Autodesk Inventor part; units mm, degrees
ref_plane "YZ Plane" through (0, 0, 0) normal (1, 0, 0) x (0, 1, 0)
ref_plane "XZ Plane" through (0, 0, 0) normal (0, 1, 0) x (-1, 0, 0)
ref_plane "XY Plane" through (0, 0, 0) normal (0, 0, 1) x (1, 0, 0)
sketch "Skizze1" plane through (0, 0, 0) normal (0, 1, 0) x (-1, 0, 0)
  line L0 (50.25, 43.85) -> (-50.25, 43.85)
  line L1 (-58.25, 35.85) -> (-58.25, -35.85)
  line L2 (-50.25, -43.85) -> (50.25, -43.85)
  line L3 (58.25, -35.85) -> (58.25, 35.85)
  line L4 (58.25, 43.85) -> (-58.25, -43.85) construction
  line L5 (-58.25, 43.85) -> (58.25, -43.85) construction
  arc A0 (58.25, 35.85) -> (50.25, 43.85) centre (50.25, 35.85) ccw
  arc A1 (50.25, -43.85) -> (58.25, -35.85) centre (50.25, -35.85) ccw
  arc A2 (-58.25, -35.85) -> (-50.25, -43.85) centre (-50.25, -35.85) ccw
  arc A3 (-50.25, 43.85) -> (-58.25, 35.85) centre (-50.25, 35.85) ccw
  point P0 (0, 0)
  dimension "d0" = 116.5
  dimension "d1" = 87.7
  dimension "d2" = 8
extrude "Extrusion1" add sketch "Skizze1" along normal blind 21
sketch "Skizze2" plane through (0, 0, 0) normal (0, -1, 0) x (1, 0, 0)
  arc A0 (58.25, 35.85) -> (50.25, 43.85) centre (50.25, 35.85) ccw
  line L0 (-50.25, 43.85) -> (50.25, 43.85)
  arc A1 (-50.25, 43.85) -> (-58.25, 35.85) centre (-50.25, 35.85) ccw
  line L1 (-58.25, -35.85) -> (-58.25, 35.85)
  arc A2 (-58.25, -35.85) -> (-50.25, -43.85) centre (-50.25, -35.85) ccw
  line L2 (50.25, -43.85) -> (-50.25, -43.85)
  arc A3 (50.25, -43.85) -> (58.25, -35.85) centre (50.25, -35.85) ccw
  line L3 (58.25, 35.85) -> (58.25, -35.85)
  line L4 (50.25, -43.85) -> (-50.25, -43.85)
  line L5 (-5.75, -43.85) -> (-5.75, 43.85)
  point P0 (0, 0)
  dimension "d5" = 64
extrude "Extrusion2" add sketch "Skizze2" along normal blind 0.1 contours L3 A3 L2 L5 L0 A0
sketch "Skizze3" plane through (0, 21, 0) normal (0, 1, 0) x (1, 0, 0)
  line L0 (-40.25, -30.75) -> (-2.65, -30.75)
  line L1 (-2.65, -30.75) -> (-2.65, 33.55)
  line L2 (-2.65, 33.55) -> (-40.25, 33.55)
  line L3 (-40.25, 33.55) -> (-40.25, -30.75)
  line L4 (-40.25, -30.75) -> (-2.65, 33.55) construction
  line L5 (-2.65, -30.75) -> (-40.25, 33.55) construction
  line L6 (-50.25, -43.85) -> (50.25, -43.85)
  line L7 (50.25, 43.85) -> (-50.25, 43.85)
  line L8 (-58.25, 35.85) -> (-58.25, -35.85)
  point P0 (0, 0)
  point P1 (-21.45, 1.4)
  dimension "d8" = 37.6
  dimension "d9" = 64.3
  dimension "d10" = 13.1
  dimension "d11" = 10.3
  dimension "d12" = 18
extrude "Extrusion3" add sketch "Skizze3" along normal blind 9
sketch "Skizze4" plane through (0, -0.1, 0) normal (0, -1, 0) x (1, 0, 0)
  line L0 (50.25, 43.85) -> (-5.75, 43.85)
  line L1 (-5.75, 43.85) -> (-5.75, -43.85)
  line L2 (-5.75, -43.85) -> (50.25, -43.85)
  arc A0 (50.25, -43.85) -> (58.25, -35.85) centre (50.25, -35.85) ccw
  line L3 (58.25, -35.85) -> (58.25, 35.85)
  arc A1 (58.25, 35.85) -> (50.25, 43.85) centre (50.25, 35.85) ccw
  line L4 (-5.75, -43.85) -> (-5.75, 43.85)
  line L5 (-50.25, 43.85) -> (-5.75, 43.85)
  arc A2 (-50.25, 43.85) -> (-58.25, 35.85) centre (-50.25, 35.85) ccw
  line L6 (-58.25, -35.85) -> (-58.25, 35.85)
  arc A3 (-58.25, -35.85) -> (-50.25, -43.85) centre (-50.25, -35.85) ccw
  line L7 (-5.75, -43.85) -> (-50.25, -43.85)
  circle A4 centre (43.75, -36.9) radius 1.1
  circle A5 centre (43.75, 29.95) radius 1.1
  circle A6 centre (-11.95, -35.9681) radius 1.1
  circle A7 centre (-8.45, 34.0319) radius 1.1
  circle A8 centre (-47.95, -34.8429) radius 1.1
  circle A9 centre (-53.15, 31.6571) radius 1.1
  point P0 (0, 0)
  dimension "d15" = 2.2
  dimension "d16" = 2.2
  dimension "d17" = 2.2
  dimension "d18" = 2.2
  dimension "d19" = 2.2
  dimension "d20" = 2.2
  dimension "d21" = 0
  dimension "d22" = 66.85
  dimension "d23" = 70
  dimension "d24" = 66.5
  dimension "d25" = 52.2
  dimension "d26" = 44.7
  dimension "d27" = 36
  dimension "d28" = 55.7
  dimension "d29" = 118.7
  dimension "d30" = 112.2809
  dimension "d31" = 86.3
  dimension "d32" = 88.0691
  dimension "d33" = 79.3976
  dimension "d34" = 13.9
  dimension "d35" = 6.95
  dimension "d36" = 14.5
  dimension "d37" = 9.8181
  dimension "d38" = 7.8819
  dimension "d39" = 9.0071
  dimension "d40" = 12.1929
  dimension "d41" = 5.1
hole "Bohrung1" at (-11.95, -0.1, -35.9681) at (-47.95, -0.1, -34.8429) at (-53.15, -0.1, 31.6571) at (-8.45, -0.1, 34.0319) at (43.75, -0.1, 29.95) at (43.75, -0.1, -36.9) direction (0, 1, 0) diameter 2 end through all
sketch "Skizze5" plane through (-58.25, 0, -35.85) normal (-1, 0, 0) x (0, 0, 1)
  line L0 (0, 0) -> (71.7, 0)
  line L1 (71.7, 0) -> (71.7, 21)
  line L2 (0, 21) -> (71.7, 21)
  line L3 (0, 0) -> (0, 21)
  line L4 (14.13, 18.35) -> (7.13, 18.35)
  line L5 (6.13, 17.35) -> (6.13, 16.05)
  line L6 (7.13, 15.05) -> (14.13, 15.05)
  line L7 (15.13, 16.05) -> (15.13, 17.35)
  arc A0 (15.13, 17.35) -> (14.13, 18.35) centre (14.13, 17.35) ccw
  arc A1 (14.13, 15.05) -> (15.13, 16.05) centre (14.13, 16.05) ccw
  arc A2 (6.13, 16.05) -> (7.13, 15.05) centre (7.13, 16.05) ccw
  arc A3 (7.13, 18.35) -> (6.13, 17.35) centre (7.13, 17.35) ccw
  line L8 (-8, 0) -> (0, 0)
  line L9 (0, 0) -> (0, 21)
  line L10 (-8, 21) -> (0, 21)
  line L11 (-8, 0) -> (-8, 21)
  point P0 (35.85, 0)
  point P1 (6.13, 15.05)
  point P2 (6.13, 18.35)
  point P3 (15.13, 15.05)
  point P4 (6.13, 16.7)
  dimension "d49" = 9
  dimension "d50" = 3.3
  dimension "d51" = 1
  dimension "d52" = 15.05
  dimension "d53" = 14.13
extrude "Extrusion4" cut sketch "Skizze5" against normal blind 6 contours A0 L7 A1 L6 A2 L5 A3 L4
equation "\"d16\" = d15"
equation "\"d17\" = d15"
equation "\"d18\" = d15"
equation "\"d19\" = d15"
equation "\"d20\" = d15"
properties part number "Isdt"
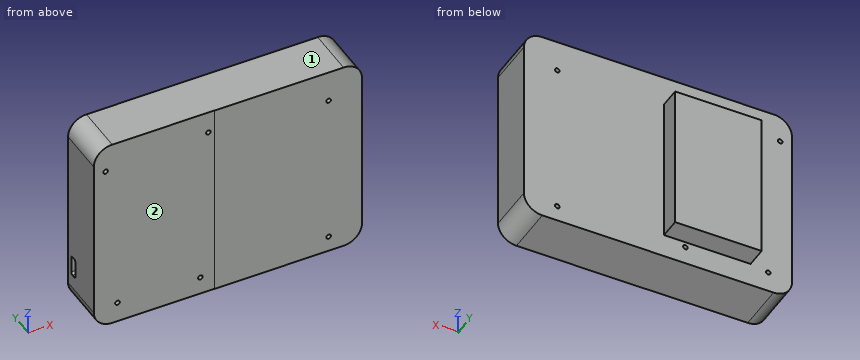
Geometry: final body of the model. Coordinates: model frame, mm. Face numbers are marked on the shaded views. A direction names the side the tool comes from. Round coordinates to 2 decimals unless told otherwise and drop trailing zeros. Write each loop counter-clockwise with the first axis right and the second up, starting at its lowest first coordinate (ties: lowest second). Pieces come first, ordered by that corner, then holes. Notation, with made-up numbers: M 15.5,52.5 L 54.5,52.5 A5 ccw 54.5,57.5 Z; hole C -32.5,58 d6. An arc over 180 degrees is marked long. Answer in a Markdown table with one row per item. Add a question column.
(1) Ray query, L1, parallel to Z at x = -11.95, y = 16.5; L2, parallel to Y at x = 6, z = -11; L3, parallel to Y at x = -32, z = 31. Return the intervals inside material, ascending.
(2) Cut plane C-C, the plane x = 7. Return the cut outline in (y, z).
(3) Reachability of the marked faces 1 and 2 from +Z, -Z, +X, -X, +Y, -Y: full face, straight path, thin tool, end or side. Return the list, or none.
(4) Cut plane B-B, the plane x = -25. Return the cut outline in (y, z), then the cut area to 3 significant figures.
(5) Contact query for flat-ended pins moving along their axis: pin 1 (5 mm diameter, centred on x = -45.5, z = -4, fed in from +Y); pin 2 (1.2 mm diameter, centred on x = 43.75, z = 29.95, fed in from -Y); pin 3 (8 mm diameter, centred on x = -16, z = 4.5, fed in from -Y); pin 4 (1.4 mm diameter, centred on x = -54, y = 16.5, fed in from -Z). Output: stop coordinate, or through.
(6) Cut plane A-A, the plane z = -6.5. Return the cut outline in (x, y), then the cut area to 3 significant figures.
Established:
| question | item | result |
|---|---|---|
| 1 | L1 | -43.85 to -36.97, -34.97 to 43.85 |
| 1 | L2 | -0.1 to 21 |
| 1 | L3 | 0 to 21 |
| 2 | outline | M -0.1,-43.85 L 21,-43.85 L 21,43.85 L -0.1,43.85 Z |
| 3 | face 1 | +Z, +X, -X, +Y, -Y |
| 3 | face 2 | +Z, -Z, -X, -Y |
| 4 | outline | M 0,-43.85 L 21,-43.85 L 21,-33.55 L 30,-33.55 L 30,30.75 L 21,30.75 L 21,43.85 L 0,43.85 Z |
| 4 | area | 2,420 mm² |
| 5 | pin 1 | y = 21 |
| 5 | pin 2 | through |
| 5 | pin 3 | y = 0 |
| 5 | pin 4 | z = -43.25 |
| 6 | outline | M -58.25,0 L -5.75,0 L -5.75,-0.1 L 58.25,-0.1 L 58.25,21 L -2.65,21 L -2.65,30 L -40.25,30 L -40.25,21 L -58.25,21 Z |
| 6 | area | 2,790 mm² |
